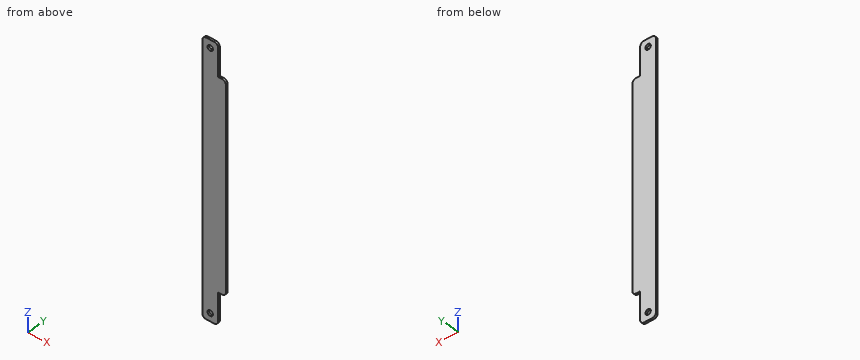
```python
from build123d import *

# Parameters (mm, degrees)
SKETCH1_R           = 2.1828125
BOSS_EXTRUDE1_DEPTH = 1.5875


with BuildPart() as part:
    # Sketch1 → Boss-Extrude1 (new body)
    with BuildSketch(Plane(origin=(0, 0, 0), x_dir=(1, 0, 0), z_dir=(0, 1, 0))):
        with BuildLine():
            Line((0, 3.175), (0, 212.725))
            ThreePointArc((0, 212.725), (0.92993597, 214.97006403), (3.175, 215.9))
            Line((3.175, 215.9), (9.525, 215.9))
            ThreePointArc((9.525, 215.9), (11.77006403, 214.97006403), (12.7, 212.725))
            Line((12.7, 212.725), (12.7, 190.5))
            Line((12.7, 190.5), (15.875, 190.5))
            ThreePointArc((15.875, 190.5), (18.12006403, 189.57006403), (19.05, 187.325))
            Line((19.05, 187.325), (19.05, 28.575))
            ThreePointArc((19.05, 28.575), (18.12006403, 26.32993597), (15.875, 25.4))
            Line((15.875, 25.4), (12.7, 25.4))
            Line((12.7, 25.4), (12.7, 3.175))
            ThreePointArc((12.7, 3.175), (11.77006403, 0.92993597), (9.525, 0))
            Line((9.525, 0), (3.175, 0))
            ThreePointArc((3.175, 0), (0.92993597, 0.92993597), (0, 3.175))
        make_face()
        with Locations((6.35, 209.55)):
            Circle(SKETCH1_R, mode=Mode.SUBTRACT)
        with Locations((6.35, 6.35)):
            Circle(SKETCH1_R, mode=Mode.SUBTRACT)
    extrude(amount=BOSS_EXTRUDE1_DEPTH)


solid = part.part
```
Verification items for the finished model (mm, model axes). Coordinates: 2 decimals unless noted, no trailing zeros. Loops run counter-clockwise (first coordinate to the right, second up) from the corner with the lowest first, then second, coordinate; pieces in that order, holes last. Notation, with made-up numbers: (69.5, 40.5) - (90.5, 40.5) arc R37 cw to (90.5, 79.5) - close; hole circle Ø8 at (84.5, -24.75). An arc over 180 degrees is marked (long way). Put each result on its own line as item: value.
Item 1: Section check A-A (z = -209.55). Enter the section's corners in (x, y).
Conclusion:
outline: (0, 0) - (4.17, 0) - (4.17, 1.59) - (0, 1.59) - close; (8.53, 0) - (12.7, 0) - (12.7, 1.59) - (8.53, 1.59) - close
Item 2: Section check B-B (y = 1.1). Enter the section's corners in (x, z) (3 decimals), then the cut area to 3 significant figures.
Conclusion:
outline: (0, -212.725) arc R3.175 ccw to (3.175, -215.9) - (9.525, -215.9) arc R3.175 ccw to (12.7, -212.725) - (12.7, -190.5) - (15.875, -190.5) arc R3.175 ccw to (19.05, -187.325) - (19.05, -28.575) arc R3.175 ccw to (15.875, -25.4) - (12.7, -25.4) - (12.7, -3.175) arc R3.175 ccw to (9.525, 0) - (3.175, 0) arc R3.175 ccw to (0, -3.175) - close; hole circle Ø4.366 at (6.35, -209.55); hole circle Ø4.366 at (6.35, -6.35)
area: 3,750 mm2
Item 3: Section check C-C (x = 6.35). Enter the section's corners in (y, z), then the cut area to 3 significant figures.
Conclusion:
outline: (0, -215.9) - (1.59, -215.9) - (1.59, -211.73) - (0, -211.73) - close; (0, -207.37) - (1.59, -207.37) - (1.59, -8.53) - (0, -8.53) - close; (0, -4.17) - (1.59, -4.17) - (1.59, 0) - (0, 0) - close
area: 329 mm2
Item 4: Scan lines: line 1 along Z through (x, y) = (6.35, 0.3); line 2 along X through (y, z) = (0.7, -209.55); line 3 along Z through (x, y) = (7.5, 0.6). Record each from-to range of solid material in increasing order.
Conclusion:
line 1: z = -215.9 to -211.73, -207.37 to -8.53, -4.17 to 0
line 2: x = 0 to 4.17, 8.53 to 12.7
line 3: z = -215.9 to -211.41, -207.69 to -8.21, -4.49 to 0
Item 5: Gauge pin test, flat end, axial feed: pin 1 Ø3.5 at (x, z) = (6.35, -209.55) entering from +Y. Record the tip position at first contact, or that the pin passes through.
Conclusion:
pin 1: passes through
